```python
from build123d import *

# Parameters (mm, degrees)
SKETCH1_R           = 54
BOSS_EXTRUDE1_DEPTH = 20.8
CUT_EXTRUDE2_START  = 2
SKETCH2_R           = 52.25
CUT_EXTRUDE2_DEPTH  = 18.8
SKETCH3_R           = 10.5
BOSS_EXTRUDE2_DEPTH = 20.8
SKETCH4_R           = 4
CUT_EXTRUDE3_DEPTH  = 2
CUT_EXTRUDE4_START  = 2
SKETCH5_W           = 13
SKETCH5_H           = 59.759182194
CUT_EXTRUDE4_DEPTH  = 18.8
SKETCH6_R           = 2
CUT_EXTRUDE5_DEPTH  = 16


with BuildPart() as part:
    # Sketch1 → Boss-Extrude1 (new body)
    with BuildSketch(Plane.XY):
        Circle(SKETCH1_R)
    extrude(amount=BOSS_EXTRUDE1_DEPTH)

    # Sketch2 → Cut-Extrude2 (cut)
    with BuildSketch(Plane.XY.offset(CUT_EXTRUDE2_START)):
        Circle(SKETCH2_R)
    extrude(amount=CUT_EXTRUDE2_DEPTH, mode=Mode.SUBTRACT)

    # Sketch3 → Boss-Extrude2 (add)
    with BuildSketch(Plane.XY):
        with BuildLine():
            ThreePointArc((-51.575187833, 16), (-54, 0), (-51.575187833, -16))
            Line((-51.575187833, -16), (-70, -16))
            ThreePointArc((-70, -16), (-86, 0), (-70, 16))
            Line((-70, 16), (-51.575187833, 16))
        make_face()
        with Locations((-70, 0)):
            Circle(SKETCH3_R, mode=Mode.SUBTRACT)
        with BuildLine():
            Line((70, 16), (51.575187833, 16))
            ThreePointArc((51.575187833, 16), (54, 0), (51.575187833, -16))
            Line((51.575187833, -16), (70, -16))
            ThreePointArc((70, -16), (86, 0), (70, 16))
        make_face()
        with Locations((70, 0)):
            Circle(SKETCH3_R, mode=Mode.SUBTRACT)
    extrude(amount=BOSS_EXTRUDE2_DEPTH)

    # Sketch4 → Cut-Extrude3 (cut)
    with BuildSketch(Plane.XY):
        Circle(SKETCH4_R)
    extrude(amount=CUT_EXTRUDE3_DEPTH, mode=Mode.SUBTRACT)

    # Sketch5 → Cut-Extrude4 (cut)
    with BuildSketch(Plane.XY.offset(CUT_EXTRUDE4_START)):
        with Locations((0, 29.879591097)):
            Rectangle(SKETCH5_W, SKETCH5_H)
    extrude(amount=CUT_EXTRUDE4_DEPTH, mode=Mode.SUBTRACT)

    # Sketch6 → Cut-Extrude5 (cut)
    with BuildSketch(Plane(origin=(0, 0, 0), x_dir=(1, 0, 0), z_dir=(0, 1, 0))):
        with Locations((-70, -10.4)):
            Circle(SKETCH6_R)
        with Locations((70, -10.4)):
            Circle(SKETCH6_R)
    extrude(amount=CUT_EXTRUDE5_DEPTH, mode=Mode.SUBTRACT)


solid = part.part
```
CAD build for the part. Positions are in the model's coordinates, mm. A direction names the side the tool comes from. Round coordinates to 2 decimals unless told otherwise and drop trailing zeros. Order: outer loops, then holes, each group sorted by start corner. A loop starts at its lowest first (then second) coordinate and runs counter-clockwise, first axis right, second up. Notation, with made-up numbers: (-13, 0.25) -> (-6, 0.25) arc R15 cw to (-6, 10.25) -> close; hole circle Ø5 at (72.5, 10). An arc over 180 degrees is marked (long way). One line per question, with ' | ' between items.
Q1. Slice it at C-C (x = 0). Write the cut outline in (y, z).
Completed:
outline: (-54, 0) -> (-4, 0) -> (-4, 2) -> (-52.25, 2) -> (-52.25, 20.8) -> (-54, 20.8) -> close; (4, 0) -> (54, 0) -> (54, 2) -> (4, 2) -> close
Q2. Two-plate mould, pull along Z, no slides. Class faces 1 (the flat face through (61, 16, 10)), 2 (the cylindrical face through (71.908, 13.111, 9.799)), 3 (the cylindrical face through (-68.092, 13.111, 9.799)), 4 (the flat face through (-1, 13, 0)): released by +Z, released by -Z, zero draft, split by the parting line, or undercut.
Completed:
face 1: zero draft | face 2: undercut | face 3: undercut | face 4: released by -Z
Q3. Probe probe 1 along X at (y, z) = (14.6, 10.4); probe 2 along X at (y, z) = (2.5, 10.75); probe 3 along Y at (x, z) = (70, 5.5). List the from-to ranges inside material, lowest first.
Completed:
probe 1: x = -76.55 to -72, -68 to -50.17, 50.17 to 68, 72 to 76.55 | probe 2: x = -85.8 to -80.2, -59.8 to -52.19, 52.19 to 59.8, 80.2 to 85.8 | probe 3: y = -16 to -10.5, 10.5 to 16
Q4. Which spindle directions (+Z, -Z, +X, -X, +Y, -Y) get a long thin tool onto all of the face, cutting with end or side? Do faces 5 (the flat face through (61, -16, 10)), 6 (the flat face through (-61, -16, 10)), 7 (the flat face through (-61, 16, 10)), 8 (the cylindrical face through (0.96, 53.99, 1.01)), 9 (the cylindrical face through (-2.206, -52.203, 11.268)). Say none if no direction does.
Completed:
face 5: +Z, -Z, +X, -Y | face 6: +Z, -Z, -X, -Y | face 7: +Z, -Z, -X, +Y | face 8: +Z, -Z, +Y | face 9: +Z
Q5. Drop flat-ended pins along their axis: pin 1 (5.5 mm diameter, centred on x = 56.5, z = 14, fed in from -Y); pin 2 (8 mm diameter, centred on x = -29, y = 10, fed in from -Z); pin 3 (4 mm diameter, centred on y = -14.5, z = 3, fed in from +X); pin 4 (5 mm diameter, centred on x = 70, z = 10.4, fed in from +Y). Give the stop position or say it passes through.
Completed:
pin 1: stops at y = -16 | pin 2: stops at z = 0 | pin 3: stops at x = 79.99 | pin 4: stops at y = 16
Q6. Slice it at D-D (x = 34.5). Write the cut outline in (y, z).
Completed:
outline: (-41.54, 0) -> (41.54, 0) -> (41.54, 20.8) -> (39.24, 20.8) -> (39.24, 2) -> (-39.24, 2) -> (-39.24, 20.8) -> (-41.54, 20.8) -> close
Q7. Slice it at A-A (z = 18). Write the cut outline in (x, y).
Completed:
outline: (-70, -16) -> (-51.58, -16) arc R54 ccw to (51.58, -16) -> (70, -16) arc R16 ccw to (70, 16) -> (51.58, 16) arc R54 ccw to (6.5, 53.61) -> (6.5, 51.84) arc R52.25 cw (long way) to (-6.5, 51.84) -> (-6.5, 53.61) arc R54 ccw to (-51.58, 16) -> (-70, 16) arc R16 ccw to start; hole circle Ø21 at (-70, 0); hole circle Ø21 at (70, 0)
Q8. Slice it at B-B (y = 0). Write the cut outline in (x, z).
Completed:
outline: (-86, 0) -> (-80.5, 0) -> (-80.5, 20.8) -> (-86, 20.8) -> close; (-59.5, 0) -> (-4, 0) -> (-4, 2) -> (-52.25, 2) -> (-52.25, 20.8) -> (-59.5, 20.8) -> close; (4, 0) -> (59.5, 0) -> (59.5, 20.8) -> (52.25, 20.8) -> (52.25, 2) -> (4, 2) -> close; (80.5, 0) -> (86, 0) -> (86, 20.8) -> (80.5, 20.8) -> close
